from build123d import *

# Parameters (mm, degrees)
F1_DEPTH = 8.636
F2_R     = 45.701569
F2_R_2   = 36.306047
F3_DEPTH = 37.338
F4_W     = 38.73572
F4_H     = 10.633336
F5_DEPTH = 29.21
F7_DEPTH = 25.4


with BuildPart() as f1:
    # F0 (on Top) → F1 (new body)
    with BuildSketch(Plane.XY):
        with BuildLine():
            Line((-7.171682, 26.046421), (-65.475807, 26.046421))
            Line((-65.475807, 26.046421), (-65.475807, -43.026961))
            Line((-65.475807, -43.026961), (12.891302, -43.026961))
            ThreePointArc((12.891302, -43.026961), (-13.155731, -13.142128), (-7.171682, 26.046421))
        make_face()
    extrude(amount=F1_DEPTH)

    # F2 (on Top) → F3 (join)
    with BuildSketch(Plane.XY):
        with Locations((27.197642, 0)):
            Circle(F2_R)
        with Locations((27.197642, 0)):
            Circle(F2_R_2, mode=Mode.SUBTRACT)
    extrude(amount=F3_DEPTH)

    # F4 (on Top) → F5 (join)
    with BuildSketch(Plane.XY):
        with Locations((-31.920592, 0.737219)):
            Rectangle(F4_W, F4_H)
    extrude(amount=F5_DEPTH)

    # F6 (on face) → F7 (cut)
    with BuildSketch(Plane.XZ.offset(4.579449)):
        Polygon((-51.288452, 8.636), (-18.27391, 29.21), (-51.288452, 29.21), align=None)
    extrude(amount=-F7_DEPTH, mode=Mode.SUBTRACT)


solid = f1.part
Can you work these out from the model? Positions are in its coordinate system, mm. A direction names the side the tool comes from. Give positions to 0.01 mm unless a question says otherwise; leave off trailing zeros. Loops run counter-clockwise (first coordinate to the right, second up) from the corner with the lowest first, then second, coordinate; pieces in that order, holes last. Notation, with made-up numbers: (1, 49.25) - (5, 49.25) arc R29 cw to (5, 82.25) - close; hole circle Ø5 at (-21.75, 68). An arc over 180 degrees is marked (long way). Answer as a JSON object with one key per item and string values.
Q1. Imagine slicing it at A-A on z = 6.5. Write out the boundary of the cut face in (x, y), plus the area to 3 significant figures.
Geometry says:
{"outline": "(-65.48, -43.03) - (11.79, -43.03) arc R45.7 ccw (long way) to (-10.36, 26.05) - (-65.48, 26.05) - close; hole circle Ø72.61 at (27.2, 0)", "area": "6,090 mm²"}
Q2. Which directions (+Z, -Z, +X, -X, +Y, -Y) give clear straight access to the entire face, cutting with the end or side of a thin tool? Please do faces 4 (the flat face through (-31, 6.054, 16)), 5 (the flat face through (-27, -43.027, 4)), 6 (the flat face through (-36, -8, 8.636)).
Geometry says:
{"face 4": "+Z, -X, +Y", "face 5": "+Z, -Z, -X, -Y", "face 6": "+Z, -X"}
Q3. If I drill on L1, parallel to Y at x = -38, z = 7; L2, parallel to Y at x = 46, z = 15.5; L3, parallel to Y at x = -23, z = 20, over which ranges is the centre line in solid material (lowest first)?
Geometry says:
{"L1": "-43.03 to 26.05", "L2": "-41.65 to -31.06, 31.06 to 41.65", "L3": "-4.58 to 6.05"}
Q4. Imagine slicing it at C-C on x = 40. Write out the boundary of the cut face in (y, z).
Geometry says:
{"outline": "(-43.87, 0) - (-33.97, 0) - (-33.97, 37.34) - (-43.87, 37.34) - close; (33.97, 0) - (43.87, 0) - (43.87, 37.34) - (33.97, 37.34) - close"}
Q5. Imagine slicing it at D-D on x = -43. Write out the boundary of the cut face in (y, z), plus the area to 3 significant figures.
Geometry says:
{"outline": "(-43.03, 0) - (26.05, 0) - (26.05, 8.64) - (6.05, 8.64) - (6.05, 13.8) - (-4.58, 13.8) - (-4.58, 8.64) - (-43.03, 8.64) - close", "area": "651 mm²"}
Q6. Imagine slicing it at B-B on y = 0. Write out the boundary of the cut face in (x, z).
Geometry says:
{"outline": "(-65.48, 0) - (-9.11, 0) - (-9.11, 37.34) - (-18.5, 37.34) - (-18.5, 29.21) - (-18.27, 29.21) - (-51.29, 8.64) - (-65.48, 8.64) - close; (63.5, 0) - (72.9, 0) - (72.9, 37.34) - (63.5, 37.34) - close"}
Q7. If we mould it in two halves opening along X, with no side actions, what happens to faces 1 (the flat face through (-38, 26.046, 4)), 2 (the cylindrical face through (70.79, 13.73, 18.41)), 3 (the cylindrical face through (-9.073, 1.596, 18.408))? For each: pulls with the +X half, pulls with the -X half, needs draft (parallel to the pull), parting line crosses it, or undercut.
Geometry says:
{"face 1": "needs draft", "face 2": "parting line crosses it", "face 3": "undercut"}
Q8. Will these pins go through, and if not, where does the flat tip stop? P1, Ø6, axis at x = 43, y = -28.5, coming from the -Z side; P2, Ø4.5, axis at x = -26, z = 2.5, coming from the -Y side; P3, Ø7, axis at x = -46.5, z = 3.5, coming from the +Y side; P4, Ø4, axis at y = 18.5, z = 33.5, coming from the +X side.
Geometry says:
{"P1": "through", "P2": "y = -43.03", "P3": "y = 26.05", "P4": "x = 69.82"}
